Here's how the part is built. I have some questions about the finished solid (model axes, mm). Face numbers are marked on the shaded views. Coordinates: 2 decimals unless noted, no trailing zeros. Loops run counter-clockwise (first coordinate to the right, second up) from the corner with the lowest first, then second, coordinate; pieces in that order, holes last. Notation, with made-up numbers: M 6,20.5 L 15,20.5 A14 ccw 15,28.5 Z; hole C 77,46 d1. An arc over 180 degrees is marked long. Use one line per item in the form item = value. Start each with the question number.
(1) Please list where these lines run through material, in increasing order: L1, parallel to Y at x = 12.75, z = 12.25; L2, parallel to Y at x = 7.75, z = 9.25; L3, parallel to Z at x = 3.25, y = 29.
(2) Will these pins go through, and if not, where does the flat tip stop? P1, Ø3.5, axis at y = 39, z = 5.5, coming from the -X side; P2, Ø5, axis at x = 18.5, y = 54.5, coming from the +Z side; P3, Ø2.5, axis at y = 39.5, z = 2, coming from the -X side.
(3) Imagine slicing it at A-A, the plane x = 10.25. Please give me the cut outline in (y, z), and give its area (3 significant figures).
(4) Imagine slicing it at C-C, the plane z = 6. Please give me the cut outline in (x, y), and give its area (3 significant figures).
(5) Imagine slicing it at B-B, the plane y = 7.5. Please give me the cut outline in (x, z).
(6) Imagine slicing it at D-D, the plane x = 20. Please give me the cut outline in (y, z).
(7) Thinking about a two-plate mould opening in Z: for the marked faces 1, 2 and 3, which applies, +Z half, -Z half, draft (parallel to the pull), parting line (faces both ways), or undercut?
```python
from build123d import *

# Parameters (mm, degrees)
F1_DEPTH  = 3
F3_DEPTH  = 10
F4_W      = 71
F4_H      = 3
F5_DEPTH  = 3
F6_W      = 23
F6_H      = 3
F7_DEPTH  = 3
F8_W      = 23
F8_H      = 3
F9_DEPTH  = 3
F10_W     = 7.5
F10_H     = 40
F11_DEPTH = 3.5
F13_DEPTH = 40
F14_DEPTH = 40


with BuildPart() as f1:
    # F0 (on Top) → F1 (new body)
    with BuildSketch(Plane.XY):
        Polygon((0, 31), (0, 0), (29, 0), (29, 77), (0, 77), (0, 52), (13, 52), (13, 31), align=None)
    extrude(amount=F1_DEPTH)

    # F2 (on face) → F3 (join)
    with BuildSketch(Plane.XY.offset(3)):
        Polygon((26, 3), (0, 3), (0, 0), (29, 0), (29, 77), (0, 77), (0, 74), (26, 74), align=None)
    extrude(amount=F3_DEPTH)

    # F4 (on face) → F5 (join)
    with BuildSketch(Plane(origin=(26, 0, 0), x_dir=(0, -1, 0), z_dir=(-1, 0, 0))):
        with Locations((-38.5, 11.5)):
            Rectangle(F4_W, F4_H)
    extrude(amount=F5_DEPTH)

    # F6 (on face) → F7 (join)
    with BuildSketch(Plane.XZ.offset(-74)):
        with Locations((11.5, 11.5)):
            Rectangle(F6_W, F6_H)
    extrude(amount=F7_DEPTH)

    # F8 (on face) → F9 (join)
    with BuildSketch(Plane(origin=(0, 3, 0), x_dir=(-1, 0, 0), z_dir=(0, 1, 0))):
        with Locations((-11.5, 11.5)):
            Rectangle(F8_W, F8_H)
    extrude(amount=F9_DEPTH)

    # F10 (on face) → F11 (join)
    with BuildSketch(Plane(origin=(0, 0, 0), x_dir=(1, 0, 0), z_dir=(0, 0, -1))):
        with Locations((20.75, -57)):
            Rectangle(F10_W, F10_H)
    extrude(amount=F11_DEPTH)

    # F12 (on face) → F13 (cut)
    with BuildSketch(Plane(origin=(0, 77, 0), x_dir=(-1, 0, 0), z_dir=(0, 1, 0))):
        Polygon((-24.5, 0), (-24.5, -3.5), (-23.5, 0), align=None)
    extrude(amount=-F13_DEPTH, mode=Mode.SUBTRACT)

    # F12 (on face) → F14 (cut)
    with BuildSketch(Plane(origin=(0, 77, 0), x_dir=(-1, 0, 0), z_dir=(0, 1, 0))):
        Polygon((-18, 0), (-17, -3.5), (-17, 0), align=None)
    extrude(amount=-F14_DEPTH, mode=Mode.SUBTRACT)


solid = f1.part
```
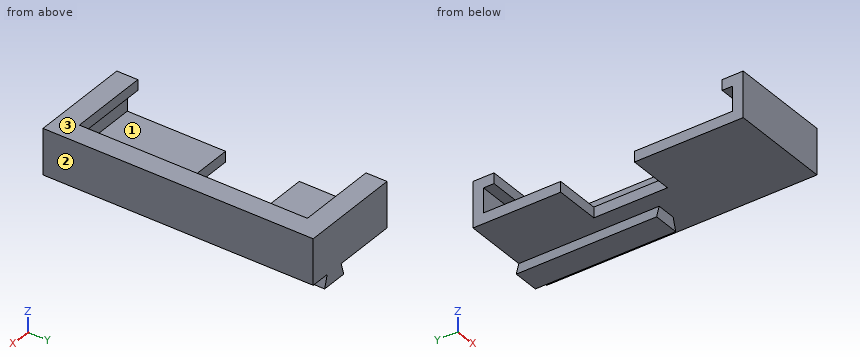
Answer:
q1.L1 = 0 to 6, 71 to 77
q1.L2 = 0 to 3, 74 to 77
q1.L3 = 0 to 3
q2.P1 = 26
q2.P2 = 3
q2.P3 = 13
q3.outline = M 0,0 L 31,0 L 31,3 L 3,3 L 3,10 L 6,10 L 6,13 L 0,13 Z; M 52,0 L 77,0 L 77,13 L 71,13 L 71,10 L 74,10 L 74,3 L 52,3 Z
q3.area = 246 mm²
q4.outline = M 0,0 L 29,0 L 29,77 L 0,77 L 0,74 L 26,74 L 26,3 L 0,3 Z
q4.area = 387 mm²
q5.outline = M 0,0 L 29,0 L 29,13 L 23,13 L 23,10 L 26,10 L 26,3 L 0,3 Z
q6.outline = M 0,0 L 37,0 L 37,-3.5 L 77,-3.5 L 77,13 L 71,13 L 71,10 L 74,10 L 74,3 L 3,3 L 3,10 L 6,10 L 6,13 L 0,13 Z
q7.face_1 = undercut
q7.face_2 = draft
q7.face_3 = +Z half
